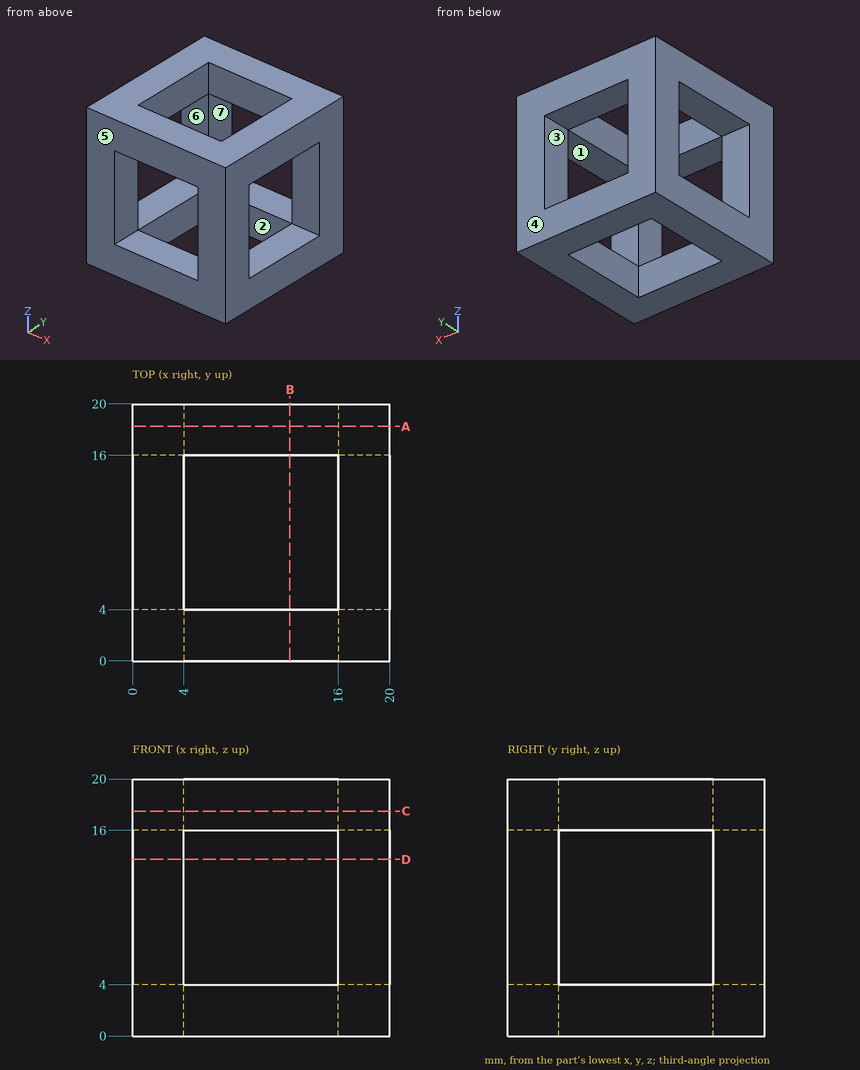
Geometry check sheet. Reference: drawing and pictorial views, mm from the part's lowest x, y, z. A direction names the side the tool comes from. Coordinates: 2 decimals unless noted, no trailing zeros. Order: outer loops, then holes, each group sorted by start corner. A loop starts at its lowest first (then second) coordinate and runs counter-clockwise, first axis right, second up. Notation, with made-up numbers: (-2, 83) -> (22, 83) arc R9 ccw to (22, 94) -> close; hole circle Ø6 at (41, -15.5). An arc over 180 degrees is marked (long way). Use CSV: the item, a comma, the result in double quotes. Start each with the question number.
Q1. Thickness scan on line 1 along X through (y, z) = (16.5, 13.5). Record the ranges inside material, lowest first.
Q2. Section check B-B, the plane x = 12.25. Record the cut outline in (y, z), and give its area (3 significant figures).
Q3. Tool access check on the marked faces 1, 2, 3, 4 and 5. Record the directions out of +Z, -Z, +X, -X, +Y, -Y that give a thin tool (end or side, any length) a straight path to the whole face; none if there is none.
Q4. Depth check by flat-ended pin: P1, Ø4, axis at x = 13.5, z = 9.5, coming from the -Y side. Enter the tip coordinate at first touch or a pass-through.
Q5. Section check A-A, the plane y = 18.25. Record the cut outline in (x, z).
Q6. Draft check along X on the marked faces 6 and 7. Enter one of: +X half, -X half, draft (parallel to the pull), parting line (faces both ways), or undercut.
Returned:
1,line 1,"x = 0 to 4, 16 to 20"
2,outline,"(0, 0) -> (4, 0) -> (4, 4) -> (0, 4) -> close; (0, 16) -> (4, 16) -> (4, 20) -> (0, 20) -> close; (16, 0) -> (20, 0) -> (20, 4) -> (16, 4) -> close; (16, 16) -> (20, 16) -> (20, 20) -> (16, 20) -> close"
2,area,"64.0 mm^2"
3,face 1,"+X, -X"
3,face 2,"+Z, -Z"
3,face 3,"+Y, -Y"
3,face 4,"+Z, -Z, +X, -X, +Y"
3,face 5,"+Z, -Z, +X, -X, -Y"
4,P1,"passes through"
5,outline,"(0, 0) -> (20, 0) -> (20, 20) -> (0, 20) -> close; hole (4, 4) -> (16, 4) -> (16, 16) -> (4, 16) -> close"
6,face 6,"draft"
6,face 7,"undercut"
